Part model, mm, in its own coordinate system. Face numbers are marked on the shaded views. Give positions to 0.01 mm unless a question says otherwise; leave off trailing zeros. Write each loop counter-clockwise with the first axis right and the second up, starting at its lowest first coordinate (ties: lowest second). Pieces come first, ordered by that corner, then holes. Notation, with made-up numbers: M 53.5,30 L 96.5,30 A20 cw 96.5,47 Z; hole C -13.75,-26 d4. An arc over 180 degrees is marked long. Use a Markdown table: item, result.
```python
from build123d import *

# Parameters (mm, degrees)
SKETCH007_R      = 1.05
EXTRUDE006_DEPTH = 20
SKETCH009_W      = 10
SKETCH009_H      = 7
EXTRUDE007_DEPTH = 5


with BuildPart() as extrude006:
    # Sketch007 → Extrude006 (new body)
    with BuildSketch(Plane(origin=(-30.396078, 0, 0), x_dir=(0, -1, 0), z_dir=(-1, 0, 0))):
        with Locations((0, 27.512153)):
            Circle(SKETCH007_R)
    extrude(amount=-EXTRUDE006_DEPTH)


with BuildPart() as extrude006_1:
    # Extrude006 placement: moved
    add(extrude006.part.moved(Location((-1, 0, 0))))


with BuildPart() as cut001:
    # Sketch009 (on Face4 of Cut) → Extrude007 (new body)
    with BuildSketch(Plane(origin=(0, 0, 30), x_dir=(1, 0, 0), z_dir=(0, 0, -1))):
        with Locations((-25.706279, 0)):
            Rectangle(SKETCH009_W, SKETCH009_H)
    extrude(amount=EXTRUDE007_DEPTH)

    # Cut001: cut Extrude006
    add(extrude006_1.part, mode=Mode.SUBTRACT)


solid = cut001.part
```
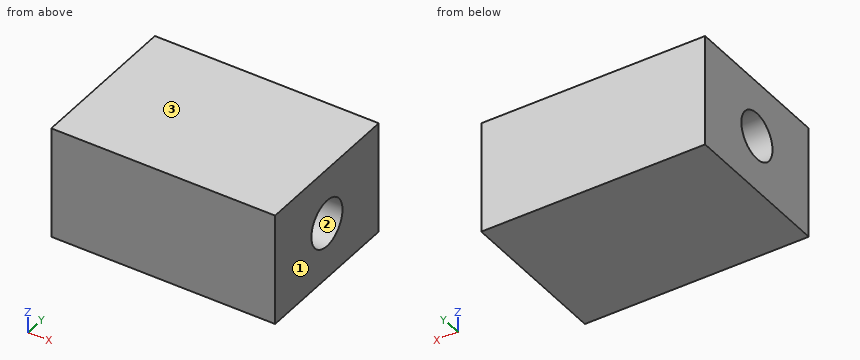
1. Cut at A-A, the plane y = 0. Give the cut face in (x, z), then the cut area to 3 significant figures.
Findings below:
| item | result |
|---|---|
| outline | M -30.71,25 L -20.71,25 L -20.71,26.46 L -30.71,26.46 Z; M -30.71,28.56 L -20.71,28.56 L -20.71,30 L -30.71,30 Z |
| area | 29.0 mm2 |
2. Two-plate mould, pull along Z, no slides. Class the marked faces 1, 2 and 3: released by +Z, released by -Z, zero draft, split by the parting line, or undercut.
Findings below:
| item | result |
|---|---|
| face 1 | zero draft |
| face 2 | undercut |
| face 3 | released by +Z |
3. Cut at B-B, the plane z = 27.85. Give the cut face in (x, y), then the cut area to 3 significant figures.
Findings below:
| item | result |
|---|---|
| outline | M -30.71,-3.5 L -20.71,-3.5 L -20.71,-0.99 L -30.71,-0.99 Z; M -30.71,0.99 L -20.71,0.99 L -20.71,3.5 L -30.71,3.5 Z |
| area | 50.1 mm2 |
4. Drill centre lines: L1, parallel to Z at x = -23, y = 0; L2, parallel to Y at x = -28.5, z = 27.25; L3, parallel to Z at x = -29, y = -0.75. Where is each one in solid material? Low to high.
Findings below:
| item | result |
|---|---|
| L1 | 25 to 26.46, 28.56 to 30 |
| L2 | -3.5 to -1.02, 1.02 to 3.5 |
| L3 | 25 to 26.78, 28.25 to 30 |
